For this review, take the finished solid that the model builds, in its own axes (mm). Round coordinates to 2 decimals unless told otherwise and drop trailing zeros. Order: outer loops, then holes, each group sorted by start corner. A loop starts at its lowest first (then second) coordinate and runs counter-clockwise, first axis right, second up. Notation, with made-up numbers: (75.5, -26) -> (131.5, -26) arc R13 cw to (131.5, -16) -> close; hole circle Ø8 at (15.25, -39.75). An arc over 180 degrees is marked (long way). Answer in a Markdown table with one row per item.
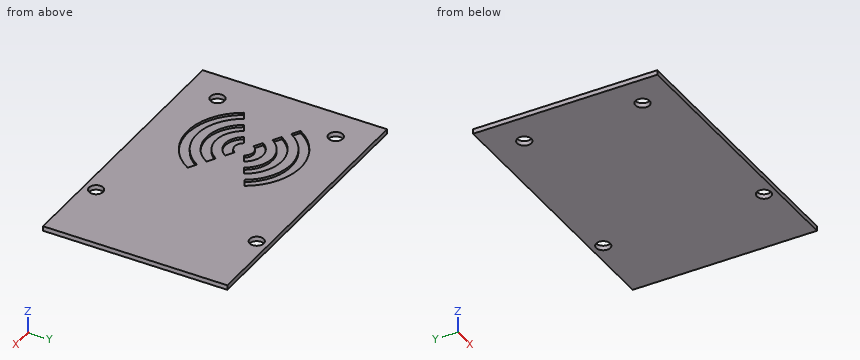
```python
from build123d import *

# Parameters (mm, degrees)
CYLINDER011_W               = 6
CYLINDER011_H               = 10
CYLINDER011_ANGLE           = 120
CYLINDER011_PLACEMENT_ANGLE = 30
CYLINDER010_W               = 8
CYLINDER010_H               = 10
CYLINDER010_ANGLE           = 120
CYLINDER010_PLACEMENT_ANGLE = 30
CYLINDER009_W               = 2
CYLINDER009_H               = 10
CYLINDER009_ANGLE           = 120
CYLINDER009_PLACEMENT_ANGLE = 30
CYLINDER008_W               = 4
CYLINDER008_H               = 10
CYLINDER008_ANGLE           = 120
CYLINDER008_PLACEMENT_ANGLE = 30
CYLINDER013_W               = 10
CYLINDER013_H               = 10
CYLINDER013_ANGLE           = 120
CYLINDER013_PLACEMENT_ANGLE = 30
CYLINDER012_W               = 12
CYLINDER012_H               = 10
CYLINDER012_ANGLE           = 120
CYLINDER012_PLACEMENT_ANGLE = 30
SKETCH003_W                 = 59
SKETCH003_H                 = 39
SKETCH003_R                 = 1.5
EXTRUDE002_DEPTH            = 1


with BuildPart() as cilindro003:
    # Cylinder011 → Cylinder011 (revolve)
    with BuildSketch(Plane.XZ):
        with Locations((3, 5)):
            Rectangle(CYLINDER011_W, CYLINDER011_H)
    revolve(axis=Axis((0, 0, 0), (0, 0, 1)), revolution_arc=CYLINDER011_ANGLE)


with BuildPart() as cilindro003_1:
    # Cylinder011 placement: moved
    add(cilindro003.part.moved(Location((-30.75, -30, 0))).rotate(Axis((-30.75, -30, 0), (0, 0, 1)), CYLINDER011_PLACEMENT_ANGLE))


with BuildPart() as obj1:
    # Cylinder010 → Cylinder010 (revolve)
    with BuildSketch(Plane.XZ):
        with Locations((4, 5)):
            Rectangle(CYLINDER010_W, CYLINDER010_H)
    revolve(axis=Axis((0, 0, 0), (0, 0, 1)), revolution_arc=CYLINDER010_ANGLE)


with BuildPart() as obj1_1:
    # Cylinder010 placement: moved
    add(obj1.part.moved(Location((-30.75, -30, 0))).rotate(Axis((-30.75, -30, 0), (0, 0, 1)), CYLINDER010_PLACEMENT_ANGLE))

    # Cut001: cut Cilindro003
    add(cilindro003_1.part, mode=Mode.SUBTRACT)


with BuildPart() as cilindro001:
    # Cylinder009 → Cylinder009 (revolve)
    with BuildSketch(Plane.XZ):
        with Locations((1, 5)):
            Rectangle(CYLINDER009_W, CYLINDER009_H)
    revolve(axis=Axis((0, 0, 0), (0, 0, 1)), revolution_arc=CYLINDER009_ANGLE)


with BuildPart() as cilindro001_1:
    # Cylinder009 placement: moved
    add(cilindro001.part.moved(Location((-30.75, -30, 0))).rotate(Axis((-30.75, -30, 0), (0, 0, 1)), CYLINDER009_PLACEMENT_ANGLE))


with BuildPart() as obj2:
    # Cylinder008 → Cylinder008 (revolve)
    with BuildSketch(Plane.XZ):
        with Locations((2, 5)):
            Rectangle(CYLINDER008_W, CYLINDER008_H)
    revolve(axis=Axis((0, 0, 0), (0, 0, 1)), revolution_arc=CYLINDER008_ANGLE)


with BuildPart() as obj2_1:
    # Cylinder008 placement: moved
    add(obj2.part.moved(Location((-30.75, -30, 0))).rotate(Axis((-30.75, -30, 0), (0, 0, 1)), CYLINDER008_PLACEMENT_ANGLE))

    # Cut: cut Cilindro001
    add(cilindro001_1.part, mode=Mode.SUBTRACT)


with BuildPart() as cilindro005:
    # Cylinder013 → Cylinder013 (revolve)
    with BuildSketch(Plane.XZ):
        with Locations((5, 5)):
            Rectangle(CYLINDER013_W, CYLINDER013_H)
    revolve(axis=Axis((0, 0, 0), (0, 0, 1)), revolution_arc=CYLINDER013_ANGLE)


with BuildPart() as cilindro005_1:
    # Cylinder013 placement: moved
    add(cilindro005.part.moved(Location((-30.75, -30, 0))).rotate(Axis((-30.75, -30, 0), (0, 0, 1)), CYLINDER013_PLACEMENT_ANGLE))


with BuildPart() as fusion:
    # Cylinder012 → Cylinder012 (revolve)
    with BuildSketch(Plane.XZ):
        with Locations((6, 5)):
            Rectangle(CYLINDER012_W, CYLINDER012_H)
    revolve(axis=Axis((0, 0, 0), (0, 0, 1)), revolution_arc=CYLINDER012_ANGLE)


with BuildPart() as fusion_1:
    # Cylinder012 placement: moved
    add(fusion.part.moved(Location((-30.75, -30, 0))).rotate(Axis((-30.75, -30, 0), (0, 0, 1)), CYLINDER012_PLACEMENT_ANGLE))

    # Cut002: cut Cilindro005
    add(cilindro005_1.part, mode=Mode.SUBTRACT)

    # Fusion: union obj1, obj2
    add(obj1_1.part)
    add(obj2_1.part)


with BuildPart() as fusion_2:
    # Fusion placement: moved
    add(fusion_1.part.moved(Location((0, 0, -6))))


with BuildPart() as obj3:
    # Part__Mirroring: instance of Fusion
    add(fusion_2.part.mirror(Plane(origin=(0, 0, 0), x_dir=(1, 0, 0), z_dir=(0, 1, 0))))


with BuildPart() as obj3_1:
    # Part__Mirroring placement: moved
    add(obj3.part.moved(Location((0, -60, 0))))

    # Fusion006: union Fusion
    add(fusion_2.part)


with BuildPart() as obj3_2:
    # Clone placement: moved
    add(obj3_1.part.moved(Location((0, 0, 9.5))))


with BuildPart() as pcb_rfid_con_logo_wifi:
    # Sketch003 → Extrude002 (new body)
    with BuildSketch(Plane.XY):
        with Locations((-20, -29.995631)):
            Rectangle(SKETCH003_W, SKETCH003_H)
        with Locations((-5.744241, -12.995631)):
            Circle(SKETCH003_R, mode=Mode.SUBTRACT)
        with Locations((-42.75, -17.482117)):
            Circle(SKETCH003_R, mode=Mode.SUBTRACT)
        with Locations((-42.75, -42.495631)):
            Circle(SKETCH003_R, mode=Mode.SUBTRACT)
        with Locations((-5.74, -46.995631)):
            Circle(SKETCH003_R, mode=Mode.SUBTRACT)
    extrude(amount=EXTRUDE002_DEPTH)


with BuildPart() as pcb_rfid_con_logo_wifi_1:
    # Extrude002 placement: moved
    add(pcb_rfid_con_logo_wifi.part.moved(Location((0, 0, 3))))

    # Cut011: cut obj3
    add(obj3_2.part, mode=Mode.SUBTRACT)


solid = pcb_rfid_con_logo_wifi_1.part
```
Q1. To check wall thickness, follow probe 1 along Y at (x, z) = (-42.75, 3.35); probe 2 along Y at (x, z) = (-39, 3.7); probe 3 along X at (y, z) = (-32.5, 3.7). State the ranges of each line that lie inside material, in increasing order.
Answer key:
| item | result |
|---|---|
| probe 1 | y = -49.5 to -44, -41 to -18.98, -15.98 to -10.5 |
| probe 2 | y = -49.5 to -38.71, -35.65 to -24.35, -21.29 to -10.5 |
| probe 3 | x = -49.5 to -33.87, -27.63 to 9.5 |
Q2. Clearance check with a flat-ended pin moving along its axis: pin 1 Ø2.5 at (x, y) = (-5.74, -47) entering from -Z. State where the tip first meets the part, or that it passes through.
Answer key:
| item | result |
|---|---|
| pin 1 | passes through |
Q3. Take a section at C-C, the plane x = -24.5. Write out the cut boundary in (y, z).
Answer key:
| item | result |
|---|---|
| outline | (-49.5, 3) -> (-10.5, 3) -> (-10.5, 4) -> (-19.76, 4) -> (-19.76, 3.5) -> (-22.19, 3.5) -> (-22.19, 4) -> (-25.01, 4) -> (-25.01, 3.5) -> (-26.39, 3.5) -> (-26.39, 4) -> (-33.61, 4) -> (-33.61, 3.5) -> (-34.99, 3.5) -> (-34.99, 4) -> (-37.81, 4) -> (-37.81, 3.5) -> (-40.24, 3.5) -> (-40.24, 4) -> (-49.5, 4) -> close |
Q4. Take a section at B-B, the plane y = -37. Write out the cut boundary in (x, z), then the cut area to 3 significant figures.
Answer key:
| item | result |
|---|---|
| outline | (-49.5, 3) -> (9.5, 3) -> (9.5, 4) -> (-21, 4) -> (-21, 3.5) -> (-23.61, 3.5) -> (-23.61, 4) -> (-26.88, 4) -> (-26.88, 3.5) -> (-34.62, 3.5) -> (-34.62, 4) -> (-37.89, 4) -> (-37.89, 3.5) -> (-40.5, 3.5) -> (-40.5, 4) -> (-49.5, 4) -> close |
| area | 52.5 mm^2 |
Q5. Take a section at A-A, the plane x = -42.75. Write out the cut boundary in (y, z), then the cut area to 3 significant figures.
Answer key:
| item | result |
|---|---|
| outline | (-49.5, 3) -> (-44, 3) -> (-44, 4) -> (-49.5, 4) -> close; (-41, 3) -> (-18.98, 3) -> (-18.98, 4) -> (-41, 4) -> close; (-15.98, 3) -> (-10.5, 3) -> (-10.5, 4) -> (-15.98, 4) -> close |
| area | 33.0 mm^2 |
